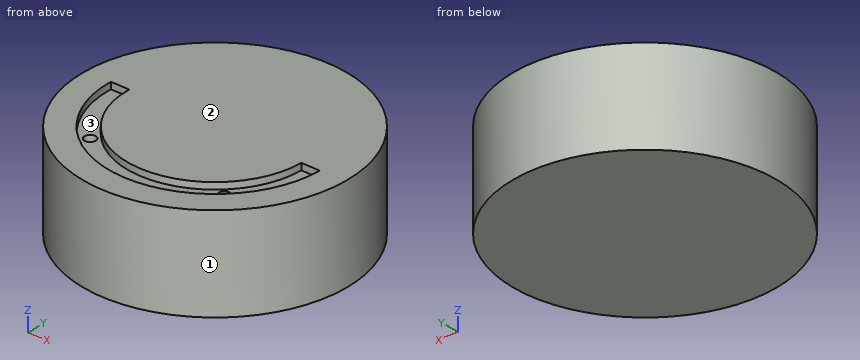
```python
from build123d import *

# Parameters (mm, degrees)
SKETCH_1_R          = 70
EXTRUDE_1_DEPTH     = 50
CUT_EXTRUDE_1_DEPTH = 3.5
SKETCH_4_R          = 3
CUT_EXTRUDE_2_DEPTH = 6


with BuildPart() as part:
    # 스케치1 → 보스-돌출1 (new body)
    with BuildSketch(Plane.XY):
        Circle(SKETCH_1_R)
    extrude(amount=EXTRUDE_1_DEPTH)

    # 스케치3 → 컷-돌출1 (cut)
    with BuildSketch(Plane.XY.offset(50)):
        with BuildLine():
            Line((-56.397174638, 0.564528852), (-46.497305932, 0.500540781))
            ThreePointArc((-46.497305932, 0.500540781), (-0.300547739, -46.499028711), (46.499891289, -0.100549136))
            Line((46.499891289, -0.100549136), (56.399759995, -0.164537207))
            ThreePointArc((56.399759995, -0.164537207), (-0.364535322, -56.39882192), (-56.397174638, 0.564528852))
        make_face()
    extrude(amount=-CUT_EXTRUDE_1_DEPTH, mode=Mode.SUBTRACT)

    # 스케치4 → 컷-돌출2 (cut)
    with BuildSketch(Plane.XY.offset(46.5)):
        with Locations((-36.040115251, -36.040115251)):
            Circle(SKETCH_4_R)
        with Locations(Location((36.040115251, -36.040115251, 0), (0, 0, 180))):
            Circle(SKETCH_4_R)
    extrude(amount=-CUT_EXTRUDE_2_DEPTH, mode=Mode.SUBTRACT)


solid = part.part
```
Read the model definition and answer for the solid it produces. Units are mm, in the model's axes. Face numbers are marked on the shaded views. Coordinates: 2 decimals unless noted, no trailing zeros. Write each loop counter-clockwise with the first axis right and the second up, starting at its lowest first coordinate (ties: lowest second). Pieces come first, ordered by that corner, then holes. Notation, with made-up numbers: (50, 38) -> (105, 38) arc R18 ccw to (105, 69) -> close; hole circle Ø6 at (88, 14.5). An arc over 180 degrees is marked (long way). Answer as a JSON object with one key per item and string values.
Q1. The part is cut by section C-C on z = 44. Give the vertices of the cut face in (x, y).
The answers:
{"outline": "circle Ø140 at (0, 0); hole circle Ø6 at (-36.04, -36.04); hole circle Ø6 at (36.04, -36.04)"}
Q2. The part is cut by section D-D on z = 22. Give the vertices of the cut face in (x, y), then the cut area to 3 significant figures.
The answers:
{"outline": "circle Ø140 at (0, 0)", "area": "15,400 mm2"}
Q3. Flat-ended cylindrical pins translate along their axes: pin 1 Ø5.5 at (x, y) = (36.04, -36.04) entering from -Z; pin 2 Ø10 at (x, z) = (-14.5, 18) entering from +Y; pin 3 Ø5 at (x, y) = (-36.04, -36.04) entering from +Z; pin 4 Ø12 at (x, z) = (7, 24) entering from +Y. Find the tip coordinate at first contact, or state that the pin passes through.
The answers:
{"pin 1": "stops at z = 0", "pin 2": "stops at y = 69.35", "pin 3": "stops at z = 40.5", "pin 4": "stops at y = 69.99"}
Q4. Determine the mould class of the marked faces 1, 2 and 3 for opening direction Y: pulls with the +Y half, pulls with the -Y half, needs draft (parallel to the pull), parting line crosses it, or undercut.
The answers:
{"face 1": "parting line crosses it", "face 2": "needs draft", "face 3": "undercut"}
Q5. The part is cut by section A-A on y = -20.5. Give the vertices of the cut face in (x, z).
The answers:
{"outline": "(-66.93, 0) -> (66.93, 0) -> (66.93, 50) -> (52.54, 50) -> (52.54, 46.5) -> (41.74, 46.5) -> (41.74, 50) -> (-41.74, 50) -> (-41.74, 46.5) -> (-52.54, 46.5) -> (-52.54, 50) -> (-66.93, 50) -> close"}
Q6. Consider line 1 (X direction, y = -11, z = 47.5); line 2 (X direction, y = 27.5, z = 21.5); line 3 (X direction, y = 57, z = 37). Determine where each line is inside the solid, lowest interval first. Write a range as [from, to].
The answers:
{"line 1": "x = [-69.13, -55.32], [-45.18, 45.18], [55.32, 69.13]", "line 2": "x = [-64.37, 64.37]", "line 3": "x = [-40.63, 40.63]"}
Q7. The part is cut by section B-B on x = 19. Give the vertices of the cut face in (y, z).
The answers:
{"outline": "(-67.37, 0) -> (67.37, 0) -> (67.37, 50) -> (-42.44, 50) -> (-42.44, 46.5) -> (-53.1, 46.5) -> (-53.1, 50) -> (-67.37, 50) -> close"}
